```python
from build123d import *

# Parameters (mm, degrees)
SKETCH_1_W           = 34
SKETCH_1_H           = 32
EXTRUDE_1_DEPTH      = 1
EXTRUDE_2_DEPTH      = 0.1
EXTRUDE_2_DEPTH_BACK = 0.05
SKETCH_2_W           = 40
SKETCH_2_H           = 6
FILLET_1_R           = 1


with BuildPart() as part:
    # 草圖1 → 填料-伸長1 (new body)
    with BuildSketch(Plane(origin=(0, 0, 0), x_dir=(1, 0, 0), z_dir=(0, 1, 0))):
        Rectangle(SKETCH_1_W, SKETCH_1_H)
    extrude(amount=EXTRUDE_1_DEPTH)

    # 草圖2 → 填料-伸長2 (add, two sides: drawn at the far end of the back side and taken through both)
    with BuildSketch(Plane(origin=(0, 0, 0), x_dir=(1, 0, 0), z_dir=(0, 1, 0)).offset(-EXTRUDE_2_DEPTH_BACK)):
        with Locations((-37, 0)):
            Rectangle(SKETCH_2_W, SKETCH_2_H)
    extrude(amount=EXTRUDE_2_DEPTH + EXTRUDE_2_DEPTH_BACK)

    # 圓角1
    fillet_1_edges = [part.edges().sort_by_distance(p)[0] for p in [
        (-17, 0.5, -16),
        (17, 0.5, -16),
        (17, 0.5, 16),
        (-17, 0.5, 16),
    ]]
    fillet(fillet_1_edges, radius=FILLET_1_R)


solid = part.part
```
Build history of the part. All positions in model axes, mm. A direction names the side the tool comes from. Round coordinates to 2 decimals unless told otherwise and drop trailing zeros. Write each loop counter-clockwise with the first axis right and the second up, starting at its lowest first coordinate (ties: lowest second). Pieces come first, ordered by that corner, then holes. Notation, with made-up numbers: (-3.75, 57) - (47.25, 57) arc R15 cw to (47.25, 83) - close; hole circle Ø11 at (81.25, 89.5). An arc over 180 degrees is marked (long way). Answer as CSV lines item,"result".
Q1. Cut at B-B (z = -5). Write the cut outline in (x, y).
Report:
outline,"(-17, 0) - (17, 0) - (17, 1) - (-17, 1) - close"
Q2. Cut at A-A (y = 0.6). Write the cut outline in (x, z).
Report:
outline,"(-17, -15) arc R1 ccw to (-16, -16) - (16, -16) arc R1 ccw to (17, -15) - (17, 15) arc R1 ccw to (16, 16) - (-16, 16) arc R1 ccw to (-17, 15) - close"
Q3. Drill centre lines: probe 1 along X at (y, z) = (0.85, -2); probe 2 along Y at (x, z) = (13.5, 12); probe 3 along Y at (x, z) = (-23, -1). Where is each one in solid material? Low to high. Write a range as [from, to].
Report:
probe 1,"x = [-17, 17]"
probe 2,"y = [0, 1]"
probe 3,"y = [-0.05, 0.1]"
Q4. Cut at C-C (x = -34.5). Write the cut outline in (y, z).
Report:
outline,"(-0.05, -3) - (0.1, -3) - (0.1, 3) - (-0.05, 3) - close"
Q5. Drop flat-ended pins along their axis: pin 1 (6 mm diameter, centred on x = -13, z = 9.5, fed in from -Y); pin 2 (3 mm diameter, centred on x = -41.5, z = 1, fed in from +Y). Give the stop position or say it passes through.
Report:
pin 1,"stops at y = 0"
pin 2,"stops at y = 0.1"
Q6. Tool access for faces 1 (the flat face through (-37, 0.1, 0)), 2 (the flat face through (0, 1, 0)): list every direction of +Z, -Z, +X, -X, +Y, -Y with a clear straight run to the whole face (end or side of a thin tool).
Report:
face 1,"+Z, -Z, -X, +Y"
face 2,"+Z, -Z, +X, -X, +Y"
